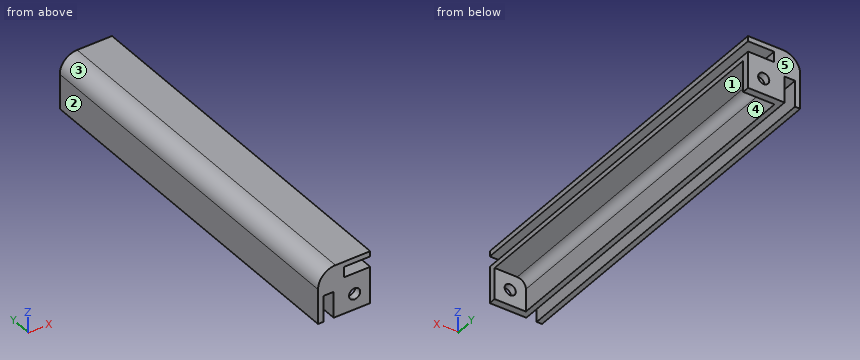
from build123d import *

# Parameters (mm, degrees)
BOSS_EXTRUDE1_DEPTH = 105
SKETCH6_R           = 1.6
BOSS_EXTRUDE2_DEPTH = 2
FILLET3_R           = 5
FILLET4_R           = 2.5
SKETCH7_R           = 1.6
BOSS_EXTRUDE3_DEPTH = 2


with BuildPart() as part:
    # Sketch4 → Boss-Extrude1 (new body)
    with BuildSketch(Plane(origin=(0, 0, 0), x_dir=(1, 0, 0), z_dir=(0, 1, 0))):
        Polygon((-7.5, -7.5), (7.5, -7.5), (7.5, -6), (0, -6), (0, -3), (7.5, -3), (7.5, -1.5), (-1.5, -1.5), (-1.5, 7.5), (-3, 7.5), (-3, 0), (-6, 0), (-6, 7.5), (-7.5, 7.5), align=None)
    extrude(amount=BOSS_EXTRUDE1_DEPTH)

    # Sketch6 → Boss-Extrude2 (add)
    with BuildSketch(Plane.XZ):
        Polygon((7.5, 7.5), (-7.5, 7.5), (-7.5, -7.5), (-6, -7.5), (-6, 0), (-3, 0), (-3, -7.5), (-1.5, -7.5), (7.5, -7.5), (7.5, 1.5), (7.5, 3), (0, 3), (0, 6), (7.5, 6), align=None)
        with Locations((3, -3)):
            Circle(SKETCH6_R, mode=Mode.SUBTRACT)
    extrude(amount=BOSS_EXTRUDE2_DEPTH)

    # Fillet3
    fillet3_edges = [part.edges().sort_by_distance(p)[0] for p in [
        (-7.5, 51.5, 7.5),
    ]]
    fillet(fillet3_edges, radius=FILLET3_R)

    # Fillet4
    fillet4_edges = [part.edges().sort_by_distance(p)[0] for p in [
        (-1.5, 52.5, 1.5),
    ]]
    fillet(fillet4_edges, radius=FILLET4_R)

    # Sketch7 → Boss-Extrude3 (add)
    with BuildSketch(Plane(origin=(0, 105, 0), x_dir=(1, 0, 0), z_dir=(0, 1, 0))):
        with BuildLine():
            Line((-1.5, 7.5), (7.5, 7.5))
            Line((7.5, 7.5), (7.5, -1.5))
            Line((7.5, -1.5), (1, -1.5))
            ThreePointArc((1, -1.5), (-0.767766953, -0.767766953), (-1.5, 1))
            Line((-1.5, 1), (-1.5, 7.5))
        make_face()
        with Locations((3, 3)):
            Circle(SKETCH7_R, mode=Mode.SUBTRACT)
    extrude(amount=-BOSS_EXTRUDE3_DEPTH)


solid = part.part
Verification items for the finished model (mm, model axes). Face numbers are marked on the shaded views. A direction names the side the tool comes from. Coordinates: 2 decimals unless noted, no trailing zeros. Write each loop counter-clockwise with the first axis right and the second up, starting at its lowest first coordinate (ties: lowest second). Pieces come first, ordered by that corner, then holes. Notation, with made-up numbers: (-16.5, -38.75) - (22.5, -38.75) arc R33 cw to (22.5, -5.75) - close; hole circle Ø1 at (-32, -26.5). An arc over 180 degrees is marked (long way). Answer as a JSON object with one key per item and string values.
(1) Tool access check on the marked faces 1 and 2. Record the directions out of +Z, -Z, +X, -X, +Y, -Y that give a thin tool (end or side, any length) a straight path to the whole face; none if there is none.
Report:
{"face 1": "-Z, +X", "face 2": "+Z, -Z, -X, +Y, -Y"}
(2) Cross-section at D-D on z = 4.25. Record the cut outline in (x, y), plus the area to 3 significant figures.
Report:
{"outline": "(-7.18, -2) - (0, -2) - (0, 105) - (-7.18, 105) - close", "area": "769 mm^2"}
(3) Cross-section at C-C on y = 12.5. Record the cut outline in (x, z), plus the area to 3 significant figures.
Report:
{"outline": "(-7.5, -7.5) - (-6, -7.5) - (-6, 0) - (-3, 0) - (-3, -7.5) - (-1.5, -7.5) - (-1.5, -1) arc R2.5 cw to (1, 1.5) - (7.5, 1.5) - (7.5, 3) - (0, 3) - (0, 6) - (7.5, 6) - (7.5, 7.5) - (-2.5, 7.5) arc R5 ccw to (-7.5, 2.5) - close", "area": "95.0 mm^2"}
(4) Cross-section at A-A on z = -3. Record the cut outline in (x, y), plus the area to 3 significant figures.
Report:
{"outline": "(-7.5, -2) - (-6, -2) - (-6, 105) - (-7.5, 105) - close; (-3, -2) - (1.4, -2) - (1.4, 0) - (-1.5, 0) - (-1.5, 103) - (1.4, 103) - (1.4, 105) - (-3, 105) - close; (4.6, -2) - (7.5, -2) - (7.5, 0) - (4.6, 0) - close; (4.6, 103) - (7.5, 103) - (7.5, 105) - (4.6, 105) - close", "area": "344 mm^2"}
(5) Thickness scan on line 1 along Z through (x, y) = (3, -1.55); line 2 along Y through (x, z) = (2, -5.5); line 3 along X through (y, z) = (104.5, -3). Record the ranges inside material, lowest first.
Report:
{"line 1": "-7.5 to -4.6, -1.4 to 3, 6 to 7.5", "line 2": "-2 to 0, 103 to 105", "line 3": "-7.5 to -6, -3 to 1.4, 4.6 to 7.5"}
(6) Cross-section at B-B on x = 3. Record the cut outline in (y, z).
Report:
{"outline": "(-2, -7.5) - (0, -7.5) - (0, -4.6) - (-2, -4.6) - close; (-2, -1.4) - (0, -1.4) - (0, 1.5) - (103, 1.5) - (103, -1.4) - (105, -1.4) - (105, 3) - (-2, 3) - close; (-2, 6) - (105, 6) - (105, 7.5) - (-2, 7.5) - close; (103, -7.5) - (105, -7.5) - (105, -4.6) - (103, -4.6) - close"}
(7) Mould release check, pull along Y, two halves, no side actions. Record for the marked faces 3, 4 and 5: pulls with the +Y half, pulls with the -Y half, needs draft (parallel to the pull), parting line crosses it, or undercut.
Report:
{"face 3": "needs draft", "face 4": "undercut", "face 5": "pulls with the +Y half"}
(8) Gauge pin test, flat ends, axial feed: pin 1 Ø2 at (y, z) = (71, -5) entering from +X; pin 2 Ø5 at (x, y) = (3.5, 92.5) entering from -Z; pin 3 Ø8 at (y, z) = (28, -4) entering from +X; pin 4 Ø3.5 at (x, z) = (3, -3) entering from +Y. Record the tip position at first contact, or that the pin passes through.
Report:
{"pin 1": "x = -1.5", "pin 2": "z = 1.5", "pin 3": "x = -1.29", "pin 4": "y = 105"}
